from build123d import *

# Parameters (mm, degrees)
F0_R     = 1.75
F1_DEPTH = 2
F2_R     = 3


with BuildPart() as f1:
    # F0 (on Top) → F1 (new body)
    with BuildSketch(Plane.XY):
        with BuildLine():
            ThreePointArc((-15.82918, -47.341641), (-14.723091, -48.551952), (-13.145898, -49))
            Line((-13.145898, -49), (-12.5, -49))
            ThreePointArc((-12.5, -49), (-10.37868, -48.12132), (-9.5, -46))
            Line((-9.5, -46), (-9.5, -35))
            ThreePointArc((-9.5, -35), (0, -25.5), (9.5, -35))
            Line((9.5, -35), (9.5, -46))
            ThreePointArc((9.5, -46), (10.37868, -48.12132), (12.5, -49))
            Line((12.5, -49), (13.145898, -49))
            ThreePointArc((13.145898, -49), (14.723091, -48.551952), (15.82918, -47.341641))
            Line((15.82918, -47.341641), (17.472136, -44.055728))
            ThreePointArc((17.472136, -44.055728), (17.866245, -42.968425), (18, -41.81966))
            Line((18, -41.81966), (18, -39.968627))
            ThreePointArc((18, -39.968627), (21.5, -36), (18, -32.031373))
            Line((18, -32.031373), (18, 21.031373))
            ThreePointArc((18, 21.031373), (21.39785, 25.898203), (16.212777, 28.787223))
            Line((16.212777, 28.787223), (12.87868, 32.12132))
            ThreePointArc((12.87868, 32.12132), (11.90541, 32.771639), (10.757359, 33))
            Line((10.757359, 33), (-10.757359, 33))
            ThreePointArc((-10.757359, 33), (-11.90541, 32.771639), (-12.87868, 32.12132))
            Line((-12.87868, 32.12132), (-16.212777, 28.787223))
            ThreePointArc((-16.212777, 28.787223), (-21.39785, 25.898203), (-18, 21.031373))
            Line((-18, 21.031373), (-18, -32.031373))
            ThreePointArc((-18, -32.031373), (-21.5, -36), (-18, -39.968627))
            Line((-18, -39.968627), (-18, -41.81966))
            ThreePointArc((-18, -41.81966), (-17.866245, -42.968425), (-17.472136, -44.055728))
            Line((-17.472136, -44.055728), (-15.82918, -47.341641))
        make_face()
        with Locations((-17.5, -36)):
            Circle(F0_R, mode=Mode.SUBTRACT)
        with BuildLine():
            ThreePointArc((-15.5, -26), (-16, -25.5), (-15.5, -25))
            Line((-15.5, -25), (-14, -25))
            ThreePointArc((-14, -25), (-13.5, -25.5), (-14, -26))
            Line((-14, -26), (-14, -29))
            ThreePointArc((-14, -29), (-13.5, -29.5), (-14, -30))
            Line((-14, -30), (-15.5, -30))
            ThreePointArc((-15.5, -30), (-16, -29.5), (-15.5, -29))
            Line((-15.5, -29), (-15.5, -26))
        make_face(mode=Mode.SUBTRACT)
        with Locations((17.5, -36)):
            Circle(F0_R, mode=Mode.SUBTRACT)
        with BuildLine():
            Line((15.5, -30), (14, -30))
            ThreePointArc((14, -30), (13.5, -29.5), (14, -29))
            Line((14, -29), (14, -26))
            ThreePointArc((14, -26), (13.5, -25.5), (14, -25))
            Line((14, -25), (15.5, -25))
            ThreePointArc((15.5, -25), (16, -25.5), (15.5, -26))
            Line((15.5, -26), (15.5, -29))
            ThreePointArc((15.5, -29), (16, -29.5), (15.5, -30))
        make_face(mode=Mode.SUBTRACT)
        with BuildLine():
            Line((-16, 17), (-16, 19))
            ThreePointArc((-16, 19), (-15, 20), (-14, 19))
            Line((-14, 19), (-14, 17))
            ThreePointArc((-14, 17), (-15, 16), (-16, 17))
        make_face(mode=Mode.SUBTRACT)
        with Locations((-17.5, 25)):
            Circle(F0_R, mode=Mode.SUBTRACT)
        with BuildLine():
            ThreePointArc((14, 19), (15, 20), (16, 19))
            Line((16, 19), (16, 17))
            ThreePointArc((16, 17), (15, 16), (14, 17))
            Line((14, 17), (14, 19))
        make_face(mode=Mode.SUBTRACT)
        with Locations((17.5, 25)):
            Circle(F0_R, mode=Mode.SUBTRACT)
    extrude(amount=F1_DEPTH)

    # F2
    f2_edges = [f1.edges().sort_by_distance(p)[0] for p in [
        (-18, -39.968627, 1),
        (-18, -32.031373, 1),
        (18, -39.968627, 1),
        (18, -32.031373, 1),
        (16.212777, 28.787223, 1),
        (18, 21.031373, 1),
        (-16.212777, 28.787223, 1),
        (-18, 21.031373, 1),
    ]]
    fillet(f2_edges, radius=F2_R)


solid = f1.part
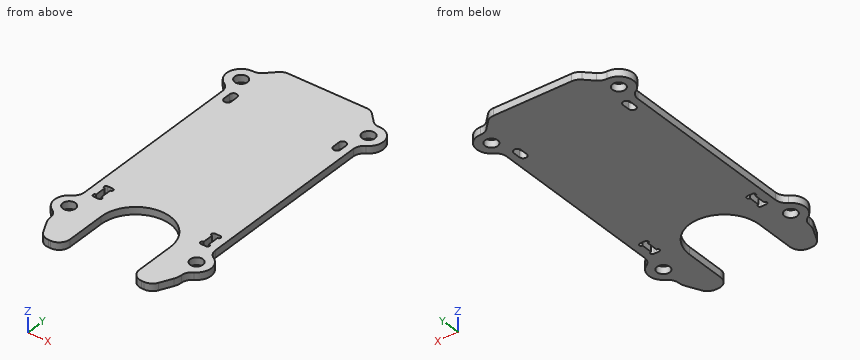
Could you check a few things on this model? Use its own coordinates, in mm. Coordinates: 2 decimals unless noted, no trailing zeros. Order: outer loops, then holes, each group sorted by start corner. A loop starts at its lowest first (then second) coordinate and runs counter-clockwise, first axis right, second up.
Q1. Will these pins go through, and if not, where does the flat tip stop? pin 1 (0.6 mm diameter, centred on y = -27, z = 1.5, fed in from +X); pin 2 (0.8 mm diameter, centred on x = 15, z = 0.5, fed in from -Y); pin 3 (0.6 mm diameter, centred on y = -27.5, z = 1.5, fed in from -X).
Q2. Suppose I cut it at B-B on x = 5.5. Please give me the cut outline in (y, z), and give its area (3 significant figures).
Q3. Suppose I cut it at C-C on y = -27. Please give me the cut outline in (x, z).
Q4. Suppose I cut it at D-D on z = 0.35. Give the number of separate pieces and of enclosed holes in the cut face, and give its area (3 significant figures).
Q5. Please list where these lines run through material, in increasing order: L1, parallel to X at y = 17.5, z = 1.6; L2, parallel to Y at x = -17.5, z = 0.6; L3, parallel to X at y = 3.5, z = 0.6.
Q6. Suppose I cut it at A-A on y = -36. Please give me the cut outline in (x, z).
Answer:
1. pin 1: stops at x = 18
1. pin 2: stops at y = -48.62
1. pin 3: stops at x = -18
2. outline: (-27.25, 0) - (33, 0) - (33, 2) - (-27.25, 2) - close
2. area: 121 mm2
3. outline: (-18, 0) - (-15.5, 0) - (-15.5, 2) - (-18, 2) - close; (-14, 0) - (-5.12, 0) - (-5.12, 2) - (-14, 2) - close; (5.12, 0) - (14, 0) - (14, 2) - (5.12, 2) - close; (15.5, 0) - (18, 0) - (18, 2) - (15.5, 2) - close
4. separate pieces: 1
4. enclosed holes: 8
4. area: 2,510 mm2
5. L1: x = -18 to -16, -14 to 14, 16 to 18
5. L2: y = -44 to -37.75, -34.25 to 23.25, 26.75 to 29
5. L3: x = -18 to 18
6. outline: (-21.5, 0) - (-19.25, 0) - (-19.25, 2) - (-21.5, 2) - close; (-15.75, 0) - (-9.5, 0) - (-9.5, 2) - (-15.75, 2) - close; (9.5, 0) - (15.75, 0) - (15.75, 2) - (9.5, 2) - close; (19.25, 0) - (21.5, 0) - (21.5, 2) - (19.25, 2) - close
